Check sheet for the modelled part. Datum: model origin and axes. Units: mm. Face numbers are marked on the shaded views. A direction names the side the tool comes from. Give positions to 0.01 mm unless a question says otherwise; leave off trailing zeros. Loops run counter-clockwise (first coordinate to the right, second up) from the corner with the lowest first, then second, coordinate; pieces in that order, holes last. Notation, with made-up numbers: (-37.75, 29.5) - (17.25, 29.5) arc R7 cw to (17.25, 41.5) - close; hole circle Ø8 at (-33, 89.5). An arc over 180 degrees is marked (long way). Use CSV: the item, a comma, the result in double quotes.
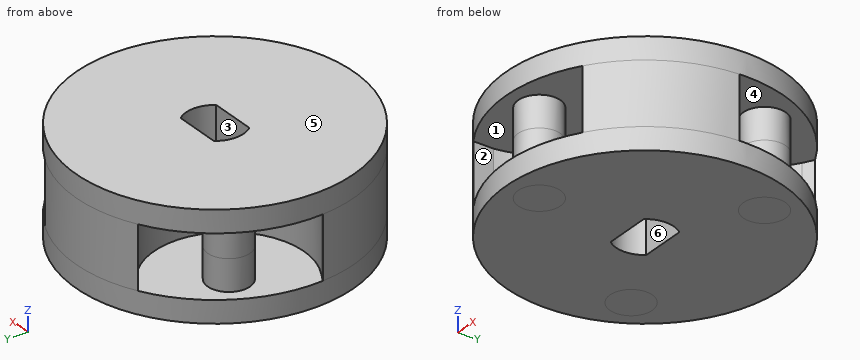
Autodesk Inventor part; units mm, degrees
ref_plane "YZ Plane" through (0, 0, 0) normal (1, 0, 0) x (0, 1, 0)
ref_plane "XZ Plane" through (0, 0, 0) normal (0, 1, 0) x (-1, 0, 0)
ref_plane "XY Plane" through (0, 0, 0) normal (0, 0, 1) x (1, 0, 0)
sketch "Skizze3" plane through (0, 0, 0) normal (0, 0, 1) x (1, 0, 0)
  circle A0 centre (82.735856, -97.364718) radius 1.5
  circle A1 centre (87.344144, -89.642424) radius 2.777622
  circle A2 centre (0, 0) radius 12.5
  line L0 (0, -9.5) -> (-8.227241, 4.75)
  line L1 (-8.227241, 4.75) -> (8.227241, 4.75)
  line L2 (8.227241, 4.75) -> (0, -9.5)
  circle A3 centre (0, -9.5) radius 1.9
  circle A4 centre (8.227241, 4.75) radius 1.9
  circle A5 centre (-8.227241, 4.75) radius 1.9
  circle A6 centre (0, 0) radius 2.6
  line L3 (-2.04939, -1.6) -> (2.04939, -1.6)
  line L4 (-2.04939, 1.6) -> (2.04939, 1.6)
  circle A7 centre (8.227241, 4.75) radius 2 construction
  dimension "d10" = 25
  dimension "d11" = 9.5
  dimension "d12" = 3.8
  dimension "d13" = 3.8
  dimension "d14" = 3.8
  dimension "d15" = 5.2
  dimension "d16" = 1.6
  dimension "d17" = 1.6
sketch "Skizze3 outline for Extrusion3" plane through (0, 0, 0) normal (0, 0, 1) x (1, 0, 0)
  circle A0 centre (0, 0) radius 12.5
  circle A1 centre (0, -9.5) radius 1.9
  arc A2 (2.04939, 1.6) -> (2.04939, -1.6) centre (0, 0) cw
  line L0 (-2.04939, 1.6) -> (2.04939, 1.6)
  arc A3 (-2.04939, -1.6) -> (-2.04939, 1.6) centre (0, 0) cw
  line L1 (2.04939, -1.6) -> (-2.04939, -1.6)
  circle A4 centre (-8.227241, 4.75) radius 1.9
  circle A5 centre (8.227241, 4.75) radius 1.9
extrude "Extrusion3" add sketch "Skizze3 outline for Extrusion3" along normal blind 2
sketch "Skizze4" plane through (0, 0, 0) normal (0, 0, -1) x (-1, 0, 0)
  circle A0 centre (0, 0) radius 12.5
  circle A1 centre (8.227241, 4.75) radius 1.9
  circle A2 centre (0, -9.5) radius 1.9
  arc A3 (-2.04939, 1.6) -> (-2.04939, -1.6) centre (0, 0) ccw
  line L0 (2.04939, 1.6) -> (-2.04939, 1.6)
  arc A4 (2.04939, -1.6) -> (2.04939, 1.6) centre (0, 0) ccw
  line L1 (-2.04939, -1.6) -> (2.04939, -1.6)
  circle A5 centre (-8.227241, 4.75) radius 1.9
  circle A6 centre (0, -9.5) radius 6.75
  circle A7 centre (-8.227241, 4.75) radius 6.75
  circle A8 centre (8.227241, 4.75) radius 6.75
  line L2 (-6.75, -16.25) -> (6.7082, -16.25)
  line L3 (6.7082, -16.25) -> (6.7082, -8.749965)
  line L4 (6.7082, -8.749965) -> (-6.75, -8.749965)
  line L5 (-6.75, -8.749965) -> (-6.75, -16.25)
  line L6 (-6.75, -16.25) -> (6.7082, -8.749965) construction
  line L7 (6.7082, -16.25) -> (-6.75, -8.749965) construction
  line L8 (5.75657, -4.470671) -> (17.447913, 2.279329)
  line L9 (17.447913, 2.279329) -> (10.697913, 13.970671)
  line L10 (10.697913, 13.970671) -> (-0.99343, 7.220671)
  line L11 (-0.99343, 7.220671) -> (5.75657, -4.470671)
  line L12 (5.75657, -4.470671) -> (10.697913, 13.970671) construction
  line L13 (17.447913, 2.279329) -> (-0.99343, 7.220671) construction
  line L14 (0, 0) -> (8.227241, 4.75)
  line L15 (8.227241, 4.75) -> (0, 0)
  line L16 (0, 0) -> (-8.263885, 4.771156)
  line L17 (-5.75657, -4.470671) -> (0.99343, 7.220671)
  line L18 (0.99343, 7.220671) -> (-10.7712, 14.012984)
  line L19 (-10.7712, 14.012984) -> (-17.5212, 2.321641)
  line L20 (-17.5212, 2.321641) -> (-5.75657, -4.470671)
  line L21 (-5.75657, -4.470671) -> (-10.7712, 14.012984) construction
  line L22 (0.99343, 7.220671) -> (-17.5212, 2.321641) construction
  point P0 (5.826917, 11.058799)
  point P1 (12.490659, -0.483141)
  point P2 (-5.826917, 11.058799)
  point P3 (-12.490659, -0.483141)
  point P4 (-6.663742, -10.575658)
  point P5 (6.663742, -10.575658)
  point P6 (-0.0209, -12.499983)
  point P7 (-11.602241, -1.095671)
  point P8 (-12.486291, -0.585265)
  point P9 (-6.75, -10.520813)
  point P10 (-6.75, -9.5)
  point P11 (6.7082, -10.547514)
  point P12 (12.486291, -0.585265)
  point P13 (11.602241, -1.095671)
  point P14 (4.852241, 10.595671)
  point P15 (5.736291, 11.106078)
  point P16 (-5.736291, 11.106078)
  point P17 (-4.852241, 10.595671)
  dimension "d20" = 13.5
  dimension "d21" = 13.5
  dimension "d22" = 13.5
sketch "Skizze4 outline for Extrusion4" plane through (0, 0, 0) normal (0, 0, -1) x (-1, 0, 0)
  line L0 (-11.602241, -1.095671) -> (-12.486291, -0.585265)
  arc A0 (-4.852241, 10.595671) -> (-11.602241, -1.095671) centre (-8.227241, 4.75) cw
  arc A1 (-12.486291, -0.585265) -> (-6.75, -10.520813) centre (0, 0) ccw
  line L1 (-5.736291, 11.106078) -> (-4.852241, 10.595671)
  line L2 (-6.75, -10.520813) -> (-6.75, -9.5)
  arc A2 (5.736291, 11.106078) -> (-5.736291, 11.106078) centre (0, 0) ccw
  arc A3 (-6.75, -9.5) -> (6.7082, -8.749965) centre (0, -9.5) cw
  line L3 (4.852241, 10.595671) -> (5.736291, 11.106078)
  line L4 (6.7082, -8.749965) -> (6.7082, -10.547514)
  arc A4 (11.602241, -1.095671) -> (4.852241, 10.595671) centre (8.227241, 4.75) cw
  arc A5 (6.7082, -10.547514) -> (12.486291, -0.585265) centre (0, 0) ccw
  line L5 (12.486291, -0.585265) -> (11.602241, -1.095671)
  arc A6 (-2.04939, -1.6) -> (-2.04939, 1.6) centre (0, 0) cw
  line L6 (2.04939, -1.6) -> (-2.04939, -1.6)
  arc A7 (2.04939, 1.6) -> (2.04939, -1.6) centre (0, 0) cw
  line L7 (-2.04939, 1.6) -> (2.04939, 1.6)
extrude "Extrusion4" add sketch "Skizze4 outline for Extrusion4" along normal blind 2.8
sketch "Skizze9" plane through (0, 0, 0) normal (0, 0, -1) x (-1, 0, 0)
  circle A0 centre (-8.227241, 4.75) radius 1.9
  circle A1 centre (8.227241, 4.75) radius 1.9
  circle A2 centre (0, -9.5) radius 1.9
  point P0 (0, 0)
sketch "Skizze9 outline for Extrusion7" plane through (0, 0, 0) normal (0, 0, -1) x (-1, 0, 0)
  circle A0 centre (0, -9.5) radius 1.9
  circle A1 centre (8.227241, 4.75) radius 1.9
  circle A2 centre (-8.227241, 4.75) radius 1.9
extrude "Extrusion7" add sketch "Skizze9 outline for Extrusion7" along normal blind 2.8 and the other way blind 2
mirror "Spiegeln1" about plane through (0, 0.976243, -2.8) normal (0, 0, -1) of "Extrusion3", "Extrusion4", "Extrusion7"
equation "\"d12\" = d13"
equation "\"d14\" = d13"
equation "\"d17\" = d16"
equation "\"d20\" = d21"
equation "\"d22\" = d21"
properties part number "Pump_Rotatio_new."
1. Set-up check for the marked faces 1, 2 and 3: record each of +Z, -Z, +X, -X, +Y, -Y from which the full face is reachable in a straight line by a thin tool's end or side.
Completed:
face 1,"none"
face 2,"-Y"
face 3,"+Z, -Z"
2. Sectioned sample at D-D, the plane y = 0. Record the boundary of the cut face in (x, z).
Completed:
outline,"(-12.5, -7.6) - (-2.6, -7.6) - (-2.6, 2) - (-12.5, 2) - (-12.5, 0) - (-3.43, 0) - (-3.43, -5.6) - (-12.5, -5.6) - close; (2.6, -7.6) - (12.5, -7.6) - (12.5, -5.6) - (3.43, -5.6) - (3.43, 0) - (12.5, 0) - (12.5, 2) - (2.6, 2) - close"
3. Release check for a two-part mould opening along Y. For the marked faces 4, 5 and 6 record: released by +Y, released by -Y, zero draft, split by the parting line, or undercut.
Completed:
face 4,"undercut"
face 5,"zero draft"
face 6,"undercut"
4. Scan lines: line 1 along Z through (x, y) = (-4.5, -6); line 2 along X through (y, z) = (-6.75, -0.5); line 3 along X through (y, z) = (3.5, -0.5). Record each from-to range of solid material in increasing order.
Completed:
line 1,"z = -7.6 to -5.6, 0 to 2"
line 2,"x = -10.52 to -6.16, 6.16 to 10.52"
line 3,"x = -9.66 to -6.8, -1.59 to 1.59, 6.8 to 9.66"
5. Sectioned sample at B-B, the plane z = -4.5. Record the boundary of the cut face in (x, y).
Completed:
outline,"(-12.49, -0.59) arc R12.5 ccw to (-6.71, -10.55) - (-6.71, -8.75) arc R6.75 cw to (6.75, -9.5) - (6.75, -10.52) arc R12.5 ccw to (12.49, -0.59) - (11.6, -1.1) arc R6.75 cw to (4.85, 10.6) - (5.74, 11.11) arc R12.5 ccw to (-5.74, 11.11) - (-4.85, 10.6) arc R6.75 cw to (-11.6, -1.1) - close; circle Ø3.8 at (-8.23, 4.75); circle Ø3.8 at (0, -9.5); circle Ø3.8 at (8.23, 4.75); hole (-2.05, -1.6) - (2.05, -1.6) arc R2.6 ccw to (2.05, 1.6) - (-2.05, 1.6) arc R2.6 ccw to start"
6. Go/stop test with flat-tipped pins: pin 1 Ø2 at (y, z) = (-9.5, -3) entering from +X; pin 2 Ø3.5 at (x, z) = (-1, -4) entering from -Y; pin 3 Ø3 at (y, z) = (5.5, 0) entering from +X. Record where each tip stops, or that it passes through.
Completed:
pin 1,"stops at x = 9.17"
pin 2,"stops at y = -12.5"
pin 3,"stops at x = 11.84"
7. Sectioned sample at A-A, the plane x = 0. Record the boundary of the cut face in (y, z), and give its area (3 significant figures).
Completed:
outline,"(-12.5, -7.6) - (-1.6, -7.6) - (-1.6, 2) - (-12.5, 2) - (-12.5, 0) - (-11.4, 0) - (-11.4, -5.6) - (-12.5, -5.6) - close; (1.6, -7.6) - (12.5, -7.6) - (12.5, 2) - (1.6, 2) - close; hole (-7.6, -5.6) - (-2.75, -5.6) - (-2.75, 0) - (-7.6, 0) - close"
area,"176 mm²"
8. Sectioned sample at C-C, the plane z = 1. Record the boundary of the cut face in (x, y), and give its area (3 significant figures).
Completed:
outline,"circle Ø25 at (0, 0); hole (-2.05, -1.6) - (2.05, -1.6) arc R2.6 ccw to (2.05, 1.6) - (-2.05, 1.6) arc R2.6 ccw to start"
area,"475 mm²"
